```python
from build123d import *

# Parameters (mm, degrees)
F0_R     = 100
F0_R_2   = 75
F0_R_3   = 25
F1_DEPTH = 12.7
F2_R     = 100
F2_R_2   = 75
F3_DEPTH = 25
F4_R     = 100
F4_R_2   = 75
F5_DEPTH = 25
F6_R     = 15


with BuildPart() as f1:
    # F0 (on Front) → F1 (new body, symmetric)
    with BuildSketch(Plane.XZ):
        Circle(F0_R)
        Circle(F0_R_2, mode=Mode.SUBTRACT)
        Circle(F0_R_2)
        Circle(F0_R_3, mode=Mode.SUBTRACT)
    extrude(amount=F1_DEPTH, both=True)

    # F2 (on face) → F3 (join)
    with BuildSketch(Plane.XZ.offset(12.7)):
        Circle(F2_R)
        Circle(F2_R_2, mode=Mode.SUBTRACT)
    extrude(amount=F3_DEPTH)

    # F4 (on face) → F5 (join)
    with BuildSketch(Plane(origin=(0, 12.7, 0), x_dir=(-1, 0, 0), z_dir=(0, 1, 0))):
        Circle(F4_R)
        Circle(F4_R_2, mode=Mode.SUBTRACT)
    extrude(amount=F5_DEPTH)

    # F6
    f6_edges = [f1.edges().sort_by_distance(p)[0] for p in [
        (100, 37.7, 0),
        (-100, -37.7, 0),
    ]]
    fillet(f6_edges, radius=F6_R)


solid = f1.part
```
Can you work these out from the model? Positions are in its coordinate system, mm. A direction names the side the tool comes from. Coordinates: 2 decimals unless noted, no trailing zeros. Order: outer loops, then holes, each group sorted by start corner. A loop starts at its lowest first (then second) coordinate and runs counter-clockwise, first axis right, second up. Notation, with made-up numbers: (56, 27.5) - (87, 27.5) arc R20 cw to (87, 48.5) - close; hole circle Ø5 at (85, 71.5). An arc over 180 degrees is marked (long way). Answer in a Markdown table with one row per item.
1. For faces 1 (the cylindrical face through (23.846, 0.178, 7.509)), 2 (the cylindrical face through (-9.764, -25.025, 74.362)), 3 (the flat face through (-18, 12.7, 18)), which set-ups out of +Z, -Z, +X, -X, +Y, -Y let a thin tool reach every point of the face, with its end or its side?
Reply:
| item | result |
|---|---|
| face 1 | +Y, -Y |
| face 2 | -Y |
| face 3 | +Y |
2. If we mould it in two halves opening along Z, with no side actions, what happens to faces 4 (the cylindrical face through (9.764, 25.025, 74.362)), 5 (the flat face through (0.4, 37.7, -75.2))? For each: pulls with the +Z half, pulls with the -Z half, needs draft (parallel to the pull), parting line crosses it, or undercut.
Reply:
| item | result |
|---|---|
| face 4 | undercut |
| face 5 | needs draft |
3. If I drill on line 1 along Z through (x, y) = (0, 7); line 2 along Z through (x, y) = (-2.5, 13.5); line 3 along X through (y, z) = (-26, -41.5), over which ranges is the centre line in solid material (lowest first)?
Reply:
| item | result |
|---|---|
| line 1 | z = -100 to -25, 25 to 100 |
| line 2 | z = -99.97 to -74.96, 74.96 to 99.97 |
| line 3 | x = -90.58 to -62.47, 62.47 to 90.58 |
4. For pin 1 (1 mm diameter, centred on y = -14.5, z = 23, fed in from -X); pin 2 (3 mm diameter, centred on y = -22, z = 26, fed in from -X); pin 3 (5 mm diameter, centred on y = -20.5, z = 18, fed in from +X), each with a flat end and sliding along its axis, tell me the tip position at first contact or that it passes through.
Reply:
| item | result |
|---|---|
| pin 1 | stops at x = -97.44 |
| pin 2 | stops at x = -96.95 |
| pin 3 | stops at x = 98.79 |
5. Suppose I cut it at B-B (z = 0). Please give me the cut outline in (x, y), and give its area (3 significant figures).
Reply:
| item | result |
|---|---|
| outline | (-100, -22.7) arc R15 ccw to (-85, -37.7) - (-75, -37.7) - (-75, -12.7) - (-25, -12.7) - (-25, 12.7) - (-75, 12.7) - (-75, 37.7) - (-85, 37.7) arc R15 ccw to (-100, 22.7) - close; (25, -12.7) - (75, -12.7) - (75, -37.7) - (85, -37.7) arc R15 ccw to (100, -22.7) - (100, 22.7) arc R15 ccw to (85, 37.7) - (75, 37.7) - (75, 12.7) - (25, 12.7) - close |
| area | 6,120 mm^2 |
6. Suppose I cut it at A-A (x = 0). Please give me the cut outline in (y, z).
Reply:
| item | result |
|---|---|
| outline | (-37.7, -85) arc R15 ccw to (-22.7, -100) - (22.7, -100) arc R15 ccw to (37.7, -85) - (37.7, -75) - (12.7, -75) - (12.7, -25) - (-12.7, -25) - (-12.7, -75) - (-37.7, -75) - close; (-37.7, 75) - (-12.7, 75) - (-12.7, 25) - (12.7, 25) - (12.7, 75) - (37.7, 75) - (37.7, 85) arc R15 ccw to (22.7, 100) - (-22.7, 100) arc R15 ccw to (-37.7, 85) - close |
7. Suppose I cut it at C-C (y = 9). Please give me the cut outline in (x, z), and give its area (3 significant figures).
Reply:
| item | result |
|---|---|
| outline | circle Ø200 at (0, 0); hole circle Ø50 at (0, 0) |
| area | 29,500 mm^2 |
